Geometry: final body of the model. Coordinates: model frame, mm. Coordinates: 2 decimals unless noted, no trailing zeros. Write each loop counter-clockwise with the first axis right and the second up, starting at its lowest first coordinate (ties: lowest second). Pieces come first, ordered by that corner, then holes.
from build123d import *

# Parameters (mm, degrees)
F0_W     = 127
F0_H     = 58.7375
F1_DEPTH = 47.625
F3_DEPTH = 47.625


with BuildPart() as f1:
    # F0 (on Front) → F1 (new body)
    with BuildSketch(Plane.XZ):
        with Locations((2.857501, -20.093455)):
            Rectangle(F0_W, F0_H)
    extrude(amount=F1_DEPTH)

    # F2 (on face) → F3 (cut)
    with BuildSketch(Plane.XZ.offset(47.625)):
        Polygon((-60.642499, 9.275295), (-60.642499, -24.062205), (-27.304999, 9.275295), align=None)
        Polygon((33.020001, 9.275295), (66.357501, -24.062205), (66.357501, 9.275295), align=None)
    extrude(amount=-F3_DEPTH, mode=Mode.SUBTRACT)


solid = f1.part
Item 1: Material intervals for probe 1 along X at (y, z) = (-39.5, 1.5); probe 2 along X at (y, z) = (-28, 3); probe 3 along Z at (x, y) = (-37, -18.5), sorted ascending.
Derived:
probe 1: x = -35.08 to 40.8
probe 2: x = -33.58 to 39.3
probe 3: z = -49.46 to -0.42
Item 2: Section B-B, the plane x = -39.5. Output: boundary loops of the cut face in (y, z) (3 decimals), plus the area to 3 significant figures.
Derived:
outline: (-47.625, -49.462) - (0, -49.462) - (0, -2.92) - (-47.625, -2.92) - close
area: 2,220 mm2
Item 3: Pin query (flat end, axial travel): pin 1 (1 mm diameter, centred on x = 27, z = -8.5, fed in from +Y); pin 2 (6 mm diameter, centred on y = -28.5, z = -12, fed in from +X). Return the tip coordinate at first contact, or that it passes through.
Derived:
pin 1: stops at y = 0
pin 2: stops at x = 57.3
Item 4: Section C-C, the plane z = -15.5. Output: boundary loops of the cut face in (x, y) (3 decimals).
Derived:
outline: (-52.08, -47.625) - (57.795, -47.625) - (57.795, 0) - (-52.08, 0) - close
Item 5: Section A-A, the plane y = -26.5. Output: boundary loops of the cut face in (x, z) (1 decimal).
Derived:
outline: (-60.6, -49.5) - (66.4, -49.5) - (66.4, -24.1) - (33, 9.3) - (-27.3, 9.3) - (-60.6, -24.1) - close
